Source: CAD feature listing. Evaluate the final solid. Frame: model axes, mm. A direction names the side the tool comes from. Give positions to 0.01 mm unless a question says otherwise; leave off trailing zeros. Loops run counter-clockwise (first coordinate to the right, second up) from the corner with the lowest first, then second, coordinate; pieces in that order, holes last. Notation, with made-up numbers: (-20.5, 51.5) -> (15.5, 51.5) arc R9 cw to (15.5, 58.5) -> close; hole circle Ø4 at (-5.5, 29). An arc over 180 degrees is marked (long way). Return JSON: item names as keys, results as strings. Group by question number.
```python
from build123d import *

# Parameters (mm, degrees)
SKETCH1_R                 = 70
BOSS_EXTRUDE2_DEPTH       = 15
SKETCH2_R                 = 65
BOSS_EXTRUDE3_DEPTH       = 3
BOSS_EXTRUDE4_DEPTH       = 5
M5X0_8_TAPPED_HOLE2_D     = 4.2
M5X0_8_TAPPED_HOLE2_DEPTH = 10
M5X0_8_TAPPED_HOLE2_TIP   = 1.2618073
SKETCH8_R                 = 3.5
CUT_EXTRUDE1_DEPTH        = 169.909563464
M5X0_8_TAPPED_HOLE3_D     = 4.2
M5X0_8_TAPPED_HOLE3_DEPTH = 10
M5X0_8_TAPPED_HOLE3_TIP   = 1.2618073
SKETCH14_R                = 3.5
CUT_EXTRUDE2_DEPTH        = 178.408330527


with BuildPart() as part:
    # Sketch1 → Boss-Extrude2 (new body)
    with BuildSketch(Plane(origin=(0, 0, 0), x_dir=(1, 0, 0), z_dir=(0, 1, 0))):
        with Locations(Location((0, 0, 0), (0, 0, 270))):
            Circle(SKETCH1_R)
    extrude(amount=BOSS_EXTRUDE2_DEPTH)

    # Sketch2 → Boss-Extrude3 (add)
    with BuildSketch(Plane.XZ):
        with Locations(Location((0, 0, 0), (0, 0, 270))):
            Circle(SKETCH2_R)
    extrude(amount=BOSS_EXTRUDE3_DEPTH)

    # Sketch3 → Boss-Extrude4 (add, symmetric)
    with BuildSketch(Plane.XY):
        with BuildLine():
            Line((-35, 62), (-35, 7))
            Line((-35, 7), (-102, 7))
            Line((-102, 7), (-119.156726544, 37.506503148))
            ThreePointArc((-119.156726544, 37.506503148), (-92.509371405, 102.772350464), (-35, 62))
        make_face()
    extrude(amount=BOSS_EXTRUDE4_DEPTH, both=True)

    # M5x0.8 Tapped Hole2
    with Locations(Plane(origin=(0, 15, 0), x_dir=(1, 0, 0), z_dir=(0, 1, 0))):
        with Locations((-23.5, 23.5), (23.5, 23.5), (23.5, -23.5), (-23.5, -23.5)):
            Hole(M5X0_8_TAPPED_HOLE2_D / 2, depth=M5X0_8_TAPPED_HOLE2_DEPTH)
            with Locations((0, 0, -(M5X0_8_TAPPED_HOLE2_DEPTH + M5X0_8_TAPPED_HOLE2_TIP / 2))):  # 118° drill point
                Cone(0, M5X0_8_TAPPED_HOLE2_D / 2, M5X0_8_TAPPED_HOLE2_TIP, mode=Mode.SUBTRACT)

    # Sketch8 → Cut-Extrude1 (cut, through all)
    with BuildSketch(Plane(origin=(0, 15, 0), x_dir=(1, 0, 0), z_dir=(0, 1, 0))):
        with Locations(Location((0, 0, 0), (0, 0, 270))):
            Circle(SKETCH8_R)
    extrude(amount=-CUT_EXTRUDE1_DEPTH, mode=Mode.SUBTRACT)

    # M5x0.8 Tapped Hole3
    with Locations(Plane(origin=(-80.46035162, 53.660377077, 5), x_dir=(1, 0, 0), z_dir=(0, 0, 1))):
        with Locations((-23.5, 23.5), (23.5, 23.5), (23.5, -23.5), (-23.5, -23.5)):
            Hole(M5X0_8_TAPPED_HOLE3_D / 2, depth=M5X0_8_TAPPED_HOLE3_DEPTH)
            with Locations((0, 0, -(M5X0_8_TAPPED_HOLE3_DEPTH + M5X0_8_TAPPED_HOLE3_TIP / 2))):  # 118° drill point
                Cone(0, M5X0_8_TAPPED_HOLE3_D / 2, M5X0_8_TAPPED_HOLE3_TIP, mode=Mode.SUBTRACT)

    # Sketch14 → Cut-Extrude2 (cut, through all)
    with BuildSketch(Plane(origin=(-80.46035162, 53.660377077, 5), x_dir=(1, 0, 0), z_dir=(0, 0, 1))):
        Circle(SKETCH14_R)
    extrude(amount=-CUT_EXTRUDE2_DEPTH, mode=Mode.SUBTRACT)


solid = part.part
```
1) Cut plane A-A on x = 0. Return loops of the section in (y, z), then the cut area to 3 significant figures.
2) Reachability of faces 5 (the face through (22.37, 9.93, -25.27)), 6 (the face through (-35, 39, 0)), 7 (the face through (-105.9, 29.36, -0.07)) from +Z, -Z, +X, -X, +Y, -Y: full face, straight path, thin tool, end or side. Return the list, or none.
3) Cut plane B-B on z = 0. Return loops of the section in (x, y).
4) Contact query for flat-ended pins moving along their axis: P1, Ø8, axis at x = -80.46, y = 53.66, coming from the -Z side; P2, Ø2, axis at x = -80.5, y = 45.5, coming from the +Z side; P3, Ø5, axis at x = -23.5, z = 23.5, coming from the +Y side. Output: stop coordinate, or through.
5) Cut plane C-C on y = 12. Return loops of the section in (x, z).
6) Cut plane D-D on z = 47. Return loops of the section in (x, y), then the cut area to 3 significant figures.
7) Mould query, pull axis Z, two halves, no side actions, for faces 1 (the face through (19.52, -1.48, -62)), 2 (the face through (-23.789, 3.957, -23.278)), 3 (the face through (-77.12, 54.71, 0.07)), 4 (the face through (-69, 56, 5)). Classes: released by +Z, released by -Z, zero draft, split by the parting line, or undercut.
8) Material intervals for line 1 (Z direction, x = -45, y = 36); line 2 (Y direction, x = -56, z = -5.5); line 3 (X direction, y = 14, z = -33), sorted ascending.
Calculated:
{
 "1": {"outline": "(-3, -65) -> (0, -65) -> (0, -70) -> (15, -70) -> (15, -3.5) -> (-3, -3.5) -> close; (-3, 3.5) -> (15, 3.5) -> (15, 70) -> (0, 70) -> (0, 65) -> (-3, 65) -> close", "area": "2,360 mm2"},
 "2": {"face 5": "+Y", "face 6": "+Z, -Z, +X, +Y", "face 7": "+Z, -Z"},
 "3": {"outline": "(-119.16, 37.51) -> (-102, 7) -> (-70, 7) -> (-70, 0) -> (-65, 0) -> (-65, -3) -> (-3.5, -3) -> (-3.5, 15) -> (-35, 15) -> (-35, 62) arc R45 ccw (long way) to start; (3.5, -3) -> (65, -3) -> (65, 0) -> (70, 0) -> (70, 15) -> (3.5, 15) -> close; hole circle Ø4.2 at (-103.96, 30.16); hole circle Ø4.2 at (-103.96, 77.16); hole circle Ø7 at (-80.46, 53.66); hole circle Ø4.2 at (-56.96, 30.16); hole circle Ø4.2 at (-56.96, 77.16)"},
 "4": {"P1": "z = -5", "P2": "z = 5", "P3": "y = 15"},
 "5": {"outline": "(-104.81, -5) -> (-69.82, -5) arc R70 ccw (long way) to (-69.82, 5) -> (-104.81, 5) -> close; hole circle Ø4.2 at (-23.5, -23.5); hole circle Ø4.2 at (-23.5, 23.5); hole circle Ø7 at (0, 0); hole circle Ø4.2 at (23.5, -23.5); hole circle Ø4.2 at (23.5, 23.5)"},
 "6": {"outline": "(-51.87, 0) -> (-44.9, 0) -> (-44.9, -3) -> (44.9, -3) -> (44.9, 0) -> (51.87, 0) -> (51.87, 15) -> (-51.87, 15) -> close", "area": "1,830 mm2"},
 "7": {"face 1": "split by the parting line", "face 2": "undercut", "face 3": "zero draft", "face 4": "released by +Z"},
 "8": {"line 1": "-5 to 5", "line 2": "-3 to 15", "line 3": "-61.73 to 61.73"}
}
